Geometry: see drawing. Coordinates: mm, zero at the bounding-box minimum. Round coordinates to 2 decimals unless told otherwise and drop trailing zeros. Order: outer loops, then holes, each group sorted by start corner. A loop starts at its lowest first (then second) coordinate and runs counter-clockwise, first axis right, second up. Notation, with made-up numbers: M 70,54 L 85,54 A11 cw 85,75 Z; hole C 85.25,-5.75 d4. An arc over 180 degrees is marked long. Answer in a Markdown table with one row per item. Add a question column.
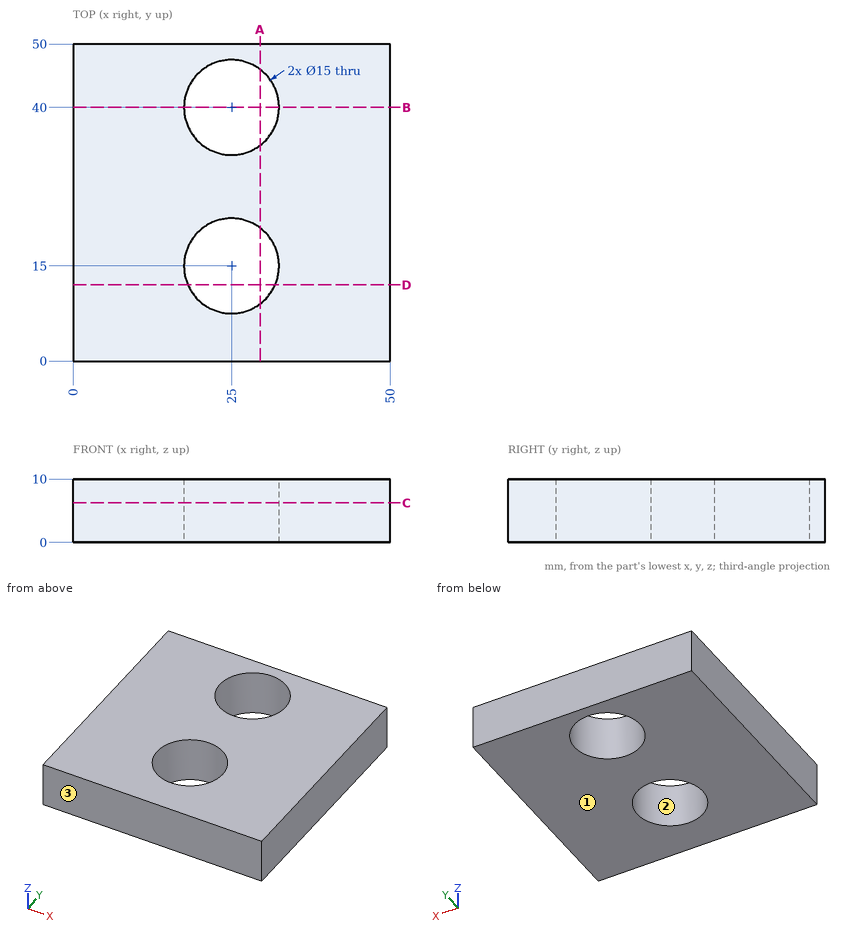
(1) Cut plane A-A (x = 29.5). Return loops of the section in (y, z), and give its area (3 significant figures).
(2) Cut plane B-B (y = 40). Return loops of the section in (x, z), and give its area (3 significant figures).
(3) Line query: line 1 (Y direction, x = 25, z = 6); line 2 (Y direction, x = 26, z = 7); line 3 (X direction, y = 44.5, z = 9.5). Output: solid intervals per line, ascending. Write a range as from..to.
(4) Cut plane C-C (z = 6.25). Return loops of the section in (x, y).
(5) Cut plane D-D (y = 12). Return loops of the section in (x, z), and give its area (3 significant figures).
(6) Draft query along Y for the marked faces 1, 2 and 3. Return one class per face: +Y half, -Y half, draft (parallel to the pull), parting line (faces both ways), or undercut.
Answer list:
| question | item | result |
|---|---|---|
| 1 | outline | M 0,0 L 9,0 L 9,10 L 0,10 Z; M 21,0 L 34,0 L 34,10 L 21,10 Z; M 46,0 L 50,0 L 50,10 L 46,10 Z |
| 1 | area | 260 mm² |
| 2 | outline | M 0,0 L 17.5,0 L 17.5,10 L 0,10 Z; M 32.5,0 L 50,0 L 50,10 L 32.5,10 Z |
| 2 | area | 350 mm² |
| 3 | line 1 | 0..7.5, 22.5..32.5, 47.5..50 |
| 3 | line 2 | 0..7.57, 22.43..32.57, 47.43..50 |
| 3 | line 3 | 0..19, 31..50 |
| 4 | outline | M 0,0 L 50,0 L 50,50 L 0,50 Z; hole C 25,15 d15; hole C 25,40 d15 |
| 5 | outline | M 0,0 L 18.13,0 L 18.13,10 L 0,10 Z; M 31.87,0 L 50,0 L 50,10 L 31.87,10 Z |
| 5 | area | 363 mm² |
| 6 | face 1 | draft |
| 6 | face 2 | undercut |
| 6 | face 3 | -Y half |
